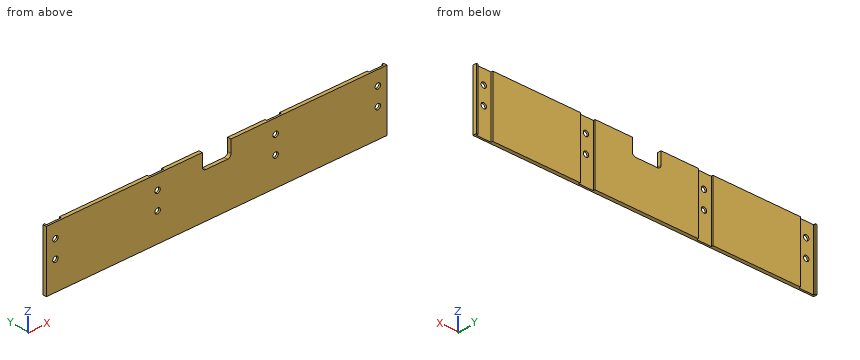
Autodesk Inventor part; units mm, degrees
ref_plane "YZ Plane" through (0, 0, 0) normal (1, 0, 0) x (0, 1, 0)
ref_plane "XZ Plane" through (0, 0, 0) normal (0, 1, 0) x (-1, 0, 0)
ref_plane "XY Plane" through (0, 0, 0) normal (0, 0, 1) x (1, 0, 0)
sketch "스케치1" plane through (0, 0, 0) normal (0, 1, 0) x (-1, 0, 0)
  line L0 (0, 0) -> (-270, 0)
  line L1 (-270, 0) -> (-270, -34)
  line L2 (-270, -34) -> (0, -34)
  line L3 (0, -34) -> (0, 0)
  dimension "d0" = 270
  dimension "d1" = 34
extrude "돌출1" add sketch "스케치1" along normal blind 2
sketch "스케치2" plane through (0, 2, 0) normal (0, 1, 0) x (1, 0, 0)
  line L0 (0, 0) -> (270, 0)
  line L1 (0, 34) -> (0, 0)
  line L2 (270, 34) -> (0, 34)
  line L3 (270, 0) -> (270, 34)
  line L4 (270, 0) -> (270, 34)
  line L5 (41, 34) -> (41, 0)
  line L6 (41, 34) -> (49.2, 34)
  line L7 (49.2, 34) -> (49.2, 0)
  line L8 (0, 0) -> (270, 0)
  line L9 (230, 34) -> (229, 34)
  line L10 (229, 34) -> (220.8, 34)
  line L11 (220.8, 34) -> (220.8, 0)
  line L12 (229, 34) -> (229, 0)
  line L13 (1, 34) -> (1, 0)
  line L14 (9.2, 34) -> (9.2, 0)
  line L15 (269, 34) -> (269, 0)
  line L16 (260.8, 34) -> (260.8, 0)
  line L17 (1, 0) -> (9.2, 0)
  line L18 (260.8, 0) -> (269, 0)
  line L19 (229, 0) -> (220.8, 0)
  line L20 (41, 0) -> (49.2, 0)
  line L21 (1, 34) -> (9.2, 34)
  line L22 (270, 34) -> (0, 34)
  line L23 (260.8, 34) -> (269, 34)
  point P0 (285, 0)
  dimension "d4" = 40
  dimension "d7" = 8.2
  dimension "d8" = 1
  dimension "d9" = 8.2
  dimension "d17" = 1
  dimension "d18" = 8.2
  dimension "d19" = 1
  dimension "d20" = 8.2
extrude "돌출4" cut sketch "스케치2" against normal blind 1 contours L13 L2 L14 L0 | L5 L2 L7 L0 | L11 L2 L12 L0 | L16 L2 L15 L0
sketch "스케치4" plane through (0, 0, 0) normal (0, -1, 0) x (1, 0, 0)
  line L0 (0, 0) -> (270, 0)
  line L1 (0, -34) -> (0, 0)
  line L2 (270, -34) -> (0, -34)
  line L3 (270, 0) -> (270, -34)
  line L4 (127, 0) -> (143, 0)
  line L5 (143, 0) -> (143, -7)
  line L6 (141, -9) -> (129, -9)
  line L7 (127, -7) -> (127, 0)
  line L8 (0, -34) -> (0, 0)
  line L9 (270, 0) -> (270, -34)
  arc A0 (127, -7) -> (129, -9) centre (129, -7) ccw
  arc A1 (141, -9) -> (143, -7) centre (141, -7) ccw
  point P0 (143, -9)
  point P1 (127, -9)
  dimension "d23" = 9
  dimension "d24" = 127
  dimension "d25" = 127
  dimension "d54" = 2
extrude "돌출5" cut sketch "스케치4" against normal blind 10 contours L0 L5 A1 L6 A0 L7
sketch "스케치5" plane through (0, 0, 0) normal (0, -1, 0) x (1, 0, 0)
  line L0 (9.2, 0) -> (1, 0)
  line L1 (9.2, -34) -> (9.2, 0)
  line L2 (1, -34) -> (9.2, -34)
  line L3 (1, 0) -> (1, -34)
  line L4 (49.2, 0) -> (41, 0)
  line L5 (49.2, -34) -> (49.2, 0)
  line L6 (41, -34) -> (49.2, -34)
  line L7 (41, 0) -> (41, -34)
  line L8 (229, 0) -> (220.8, 0)
  line L9 (229, -34) -> (229, 0)
  line L10 (220.8, -34) -> (229, -34)
  line L11 (220.8, 0) -> (220.8, -34)
  line L12 (269, 0) -> (260.8, 0)
  line L13 (269, -34) -> (269, 0)
  line L14 (260.8, -34) -> (269, -34)
  line L15 (260.8, 0) -> (260.8, -34)
  circle A0 centre (5.1, -8) radius 1.5
  circle A1 centre (5.1, -18) radius 1.5
  circle A2 centre (45.1, -8) radius 1.5
  circle A3 centre (45.1, -18) radius 1.5
  circle A4 centre (224.9, -18) radius 1.5
  circle A5 centre (224.9, -8) radius 1.5
  circle A6 centre (264.9, -8) radius 1.5
  circle A7 centre (264.9, -18) radius 1.5
  point P0 (0, 0)
  dimension "d28" = 3
  dimension "d29" = 3
  dimension "d30" = 3
  dimension "d31" = 4.1
  dimension "d32" = 4.1
  dimension "d33" = 4.1
  dimension "d34" = 4.1
  dimension "d35" = 4.1
  dimension "d36" = 4.1
  dimension "d37" = 4.1
  dimension "d38" = 4.1
  dimension "d39" = 8
  dimension "d40" = 16
  dimension "d41" = 16
  dimension "d42" = 8
  dimension "d43" = 8
  dimension "d44" = 3
  dimension "d45" = 16
  dimension "d46" = 3
  dimension "d47" = 16
  dimension "d48" = 8
  dimension "d49" = 3
  dimension "d50" = 3
  dimension "d51" = 3
extrude "돌출6" cut sketch "스케치5" against normal blind 10 contours A0 | A1 | A2 | A3 | A4 | A5 | A6 | A7
sketch "스케치6" plane through (0, 2, 0) normal (0, 1, 0) x (1, 0, 0)
  line L0 (143, 7) -> (143, 0)
  line L1 (143, 0) -> (220.8, 0)
  line L2 (220.8, 0) -> (220.8, 34)
  line L3 (220.8, 34) -> (49.2, 34)
  line L4 (49.2, 34) -> (49.2, 0)
  line L5 (127, 0) -> (127, 7)
  arc A0 (129, 9) -> (127, 7) centre (129, 7) ccw
  line L6 (129, 9) -> (141, 9)
  arc A1 (143, 7) -> (141, 9) centre (141, 7) ccw
  circle A2 centre (264.9, 8) radius 1.5
  circle A3 centre (224.9, 18) radius 1.5
  circle A4 centre (45.1, 8) radius 1.5
  circle A5 centre (5.1, 8) radius 1.5
  circle A6 centre (5.1, 18) radius 1.5
  circle A7 centre (45.1, 18) radius 1.5
  circle A8 centre (224.9, 8) radius 1.5
  circle A9 centre (264.9, 18) radius 1.5
  line L7 (143, 0) -> (143, 7)
  arc A10 (141, 9) -> (143, 7) centre (141, 7) ccw
  line L8 (141, 9) -> (129, 9)
  arc A11 (127, 7) -> (129, 9) centre (129, 7) ccw
  line L9 (127, 7) -> (127, 0)
  line L10 (0, 0) -> (127, 0)
  line L11 (0, 34) -> (0, 0)
  line L12 (270, 34) -> (0, 34)
  line L13 (270, 0) -> (270, 34)
  line L14 (49.2, 0) -> (127, 0)
  line L15 (98, 34) -> (106.2, 34)
  line L16 (106.2, 34) -> (106.2, 0)
  line L17 (106.2, 0) -> (98, 0)
  line L18 (98, 0) -> (98, 34)
  line L19 (220.8, 34) -> (49.2, 34)
  line L20 (143, 0) -> (220.8, 0)
  line L21 (163.8, 34) -> (172, 34)
  line L22 (172, 34) -> (172, 0)
  line L23 (172, 0) -> (163.8, 0)
  line L24 (163.8, 0) -> (163.8, 34)
  line L25 (229, 34) -> (229, 0)
  line L26 (229, 0) -> (260.8, 0)
  line L27 (260.8, 0) -> (260.8, 34)
  line L28 (260.8, 34) -> (229, 34)
  line L29 (41, 0) -> (41, 34)
  line L30 (41, 34) -> (9.2, 34)
  line L31 (9.2, 34) -> (9.2, 0)
  line L32 (9.2, 0) -> (41, 0)
  line L33 (1, 0) -> (1, 34)
  line L34 (1, 34) -> (0, 34)
  line L35 (0, 34) -> (0, 0)
  line L36 (0, 0) -> (1, 0)
  line L37 (269, 34) -> (269, 0)
  line L38 (269, 0) -> (270, 0)
  line L39 (270, 0) -> (270, 34)
  line L40 (270, 34) -> (269, 34)
  line L41 (49.2, 0) -> (127, 0)
  line L42 (143, 0) -> (270, 0)
  point P0 (163, 0)
  dimension "d55" = 8.2
  dimension "d56" = 8.2
  dimension "d57" = 98
  dimension "d58" = 98
extrude "돌출7" cut sketch "스케치6" against normal blind 1 contours L24 L3 L22 L1 | L16 L10 L18 L3
sketch "스케치7" plane through (0, 1, 0) normal (0, 1, 0) x (1, 0, 0)
  line L0 (106.2, 34) -> (106.2, 0)
  line L1 (98, 34) -> (106.2, 34)
  line L2 (98, 0) -> (98, 34)
  line L3 (106.2, 0) -> (98, 0)
  line L4 (172, 34) -> (172, 0)
  line L5 (163.8, 34) -> (172, 34)
  line L6 (163.8, 0) -> (163.8, 34)
  line L7 (172, 0) -> (163.8, 0)
  circle A0 centre (102.1, 8) radius 1.5
  circle A1 centre (102.1, 18) radius 1.5
  circle A2 centre (167.9, 18) radius 1.5
  circle A3 centre (167.9, 8) radius 1.5
  point P0 (0, 0)
  dimension "d61" = 3
  dimension "d62" = 3
  dimension "d63" = 3
  dimension "d64" = 3
  dimension "d65" = 4.1
  dimension "d66" = 4.1
  dimension "d67" = 4.1
  dimension "d68" = 4.1
  dimension "d69" = 8
  dimension "d71" = 8
  dimension "d75" = 16
  dimension "d76" = 16
extrude "돌출8" cut sketch "스케치7" against normal blind 1 contours A0 | A1 | A2 | A3
sketch "스케치8" plane through (0, 2, 0) normal (0, 1, 0) x (1, 0, 0)
  line L0 (230, 0) -> (230, 33)
  line L1 (40, 0) -> (40, 33)
  line L2 (230, 0) -> (270, 0)
  line L3 (270, 0) -> (270, 34)
  line L4 (270, 34) -> (230, 34)
  line L5 (230, 34) -> (230, 0)
  line L6 (1, 34) -> (0, 34)
  line L7 (40, 0) -> (0, 0)
  line L8 (0, 0) -> (0, 34)
  line L9 (0, 34) -> (40, 34)
  line L10 (40, 34) -> (40, 0)
extrude "돌출9" cut sketch "스케치8" against normal blind 10
properties part number "앞뒷판_밑" material "알루미늄 6061"
For this review, take the finished solid that the model builds, in its own axes (mm). Coordinates: 2 decimals unless noted, no trailing zeros. Order: outer loops, then holes, each group sorted by start corner. A loop starts at its lowest first (then second) coordinate and runs counter-clockwise, first axis right, second up. Notation, with made-up numbers: (35, -32) - (76, -32) arc R6 ccw to (76, -23) - close; hole circle Ø5 at (8.5, -26). An arc over 180 degrees is marked (long way). Use one line per item in the form item = value.
Q1. Consider section B-B (z = -24.5). Give the boundary of the cut face in (x, y).
Checked values:
outline = (40, 0) - (230, 0) - (230, 2) - (229, 2) - (229, 1) - (220.8, 1) - (220.8, 2) - (172, 2) - (172, 1) - (163.8, 1) - (163.8, 2) - (106.2, 2) - (106.2, 1) - (98, 1) - (98, 2) - (49.2, 2) - (49.2, 1) - (41, 1) - (41, 2) - (40, 2) - close
Q2. Consider section A-A (y = 0.65). Give the number of separate pieces and of enclosed holes in the cut face, then the cut area to 3 significant figures.
Checked values:
separate_pieces = 1
enclosed_holes = 8
area = 6,260 mm2
Q3. For P1, Ø4, axis at x = 45, z = -9, coming from the +Y side, flat-tipped, find the tip position at first contact; note if it passes through.
Checked values:
P1 = 1
Q4. For probe 1 along Z at (x, y) = (45.1, 0.3); probe 2 along X at (y, z) = (1.2, -3); probe 3 along X at (y, z) = (1.7, -27), list the stretches that pass through material, from the lowest coordinate up. Write a range as from..to.
Checked values:
probe_1 = -34..-19.5, -16.5..-9.5, -6.5..0
probe_2 = 40..41, 49.2..98, 106.2..127, 143..163.8, 172..220.8, 229..230
probe_3 = 40..41, 49.2..98, 106.2..163.8, 172..220.8, 229..230
